Autodesk Inventor part; units mm, degrees
ref_plane "YZ Plane" through (0, 0, 0) normal (1, 0, 0) x (0, 1, 0)
ref_plane "XZ Plane" through (0, 0, 0) normal (0, 1, 0) x (-1, 0, 0)
ref_plane "XY Plane" through (0, 0, 0) normal (0, 0, 1) x (1, 0, 0)
sketch "Sketch1" plane through (0, 0, 0) normal (0, 0, 1) x (1, 0, 0)
  circle A0 centre (119.5, -44.5) radius 1.5
  circle A1 centre (82.7, -44.5) radius 1.5
  circle A2 centre (44.5, -44.5) radius 1.5
  line L0 (0, 0) -> (140, 0)
  line L1 (140, 0) -> (140, -47.5)
  line L2 (140, -47.5) -> (0, -47.5)
  line L3 (0, -47.5) -> (0, 0)
  line L4 (0, -47.5) -> (20, -47.5)
  line L5 (20, -47.5) -> (20, -77.5)
  line L6 (20, -77.5) -> (0, -77.5)
  line L7 (0, -77.5) -> (0, -47.5)
  dimension "d8" = 3
  dimension "d10" = 36.8
  dimension "d11" = 75
  dimension "d15" = 140
  dimension "d16" = 47.5
  dimension "d17" = 20
  dimension "d18" = 30
extrude "Extrusion1" add sketch "Sketch1" along normal blind 2.5
properties part number "IR_PCB_Inventor"
Could you check a few things on this model? Use its own coordinates, in mm. A direction names the side the tool comes from. Give positions to 0.01 mm unless a question says otherwise; leave off trailing zeros. Loops run counter-clockwise (first coordinate to the right, second up) from the corner with the lowest first, then second, coordinate; pieces in that order, holes last. Notation, with made-up numbers: (-4, -31) -> (53, -31) arc R27 cw to (53, 3) -> close; hole circle Ø2 at (49, 36.5). An arc over 180 degrees is marked (long way). Put each result on its own line as item: value.
(1) Please list where these lines run through material, in increasing order: probe 1 along Y at (x, z) = (82.7, 1.7); probe 2 along X at (y, z) = (-45, 1.75); probe 3 along Y at (x, z) = (41.5, 0.25). Write a range as [from, to].
Computed:
probe 1: [-47.5, -46], [-43, 0]
probe 2: [0, 43.09], [45.91, 81.29], [84.11, 118.09], [120.91, 140]
probe 3: [-47.5, 0]
(2) Imagine slicing it at C-C on z = 1.75. Write out the boundary of the cut face in (x, y).
Computed:
outline: (0, -77.5) -> (20, -77.5) -> (20, -47.5) -> (140, -47.5) -> (140, 0) -> (0, 0) -> close; hole circle Ø3 at (44.5, -44.5); hole circle Ø3 at (82.7, -44.5); hole circle Ø3 at (119.5, -44.5)
(3) For faces 1 (the face through (20, -62, 1)), 2 (the face through (0, -39, 1)), which set-ups out of +Z, -Z, +X, -X, +Y, -Y let a thin tool reach every point of the face, with its end or its side?
Computed:
face 1: +Z, -Z, +X, -Y
face 2: +Z, -Z, -X, +Y, -Y
(4) Imagine slicing it at B-B on x = 44.5. Write out the boundary of the cut face in (y, z), plus the area to 3 significant figures.
Computed:
outline: (-47.5, 0) -> (-46, 0) -> (-46, 2.5) -> (-47.5, 2.5) -> close; (-43, 0) -> (0, 0) -> (0, 2.5) -> (-43, 2.5) -> close
area: 111 mm^2
(5) Imagine slicing it at D-D on x = 95.5. Write out the boundary of the cut face in (y, z), plus the area to 3 significant figures.
Computed:
outline: (-47.5, 0) -> (0, 0) -> (0, 2.5) -> (-47.5, 2.5) -> close
area: 119 mm^2
(6) Thinking about a two-plate mould opening in X: for faces 3 (the face through (140, -23, 1)), 4 (the face through (81, -47.5, 1)), 5 (the face through (118.3, -43.6, 1.2)), which applies, pulls with the +X half, pulls with the -X half, needs draft (parallel to the pull), parting line crosses it, or undercut?
Computed:
face 3: pulls with the +X half
face 4: needs draft
face 5: undercut
(7) Imagine slicing it at A-A on y = -44.5. Write out the boundary of the cut face in (x, z), plus the area to 4 significant figures.
Computed:
outline: (0, 0) -> (43, 0) -> (43, 2.5) -> (0, 2.5) -> close; (46, 0) -> (81.2, 0) -> (81.2, 2.5) -> (46, 2.5) -> close; (84.2, 0) -> (118, 0) -> (118, 2.5) -> (84.2, 2.5) -> close; (121, 0) -> (140, 0) -> (140, 2.5) -> (121, 2.5) -> close
area: 327.5 mm^2
(8) I'm going to push a flat-ended pin straight in: pin 1 Ø2.5 at (x, y) = (82.7, -44.5) entering from -Z. Where does the tip first touch, or does it pass through?
Computed:
pin 1: through
